from build123d import *

# Parameters (mm, degrees)
SKETCH1_W           = 22.5
SKETCH1_H           = 12.2
BOSS_EXTRUDE1_DEPTH = 22.3
SKETCH2_W           = 12.2
SKETCH2_H           = 2.5
BOSS_EXTRUDE2_DEPTH = 5
CUT_EXTRUDE1_DEPTH  = 28.554396191
SKETCH5_R           = 6.1
BOSS_EXTRUDE3_DEPTH = 4.25
SKETCH6_R           = 2.5
BOSS_EXTRUDE4_DEPTH = 2


with BuildPart() as part:
    # Sketch1 → Boss-Extrude1 (new body)
    with BuildSketch(Plane(origin=(0, 0, 0), x_dir=(1, 0, 0), z_dir=(0, 1, 0))):
        with Locations((3.369036145, -0.994939759)):
            Rectangle(SKETCH1_W, SKETCH1_H)
    extrude(amount=BOSS_EXTRUDE1_DEPTH)

    # Sketch2 → Boss-Extrude2 (add)
    with BuildSketch(Plane(origin=(14.619036145, 0, 0), x_dir=(0, 0, -1), z_dir=(1, 0, 0))):
        with Locations((-0.994939759, 16.75)):
            Rectangle(SKETCH2_W, SKETCH2_H)
    boss_extrude2 = extrude(amount=BOSS_EXTRUDE2_DEPTH)

    # Sketch3 → Cut-Extrude1 (cut, through all)
    with BuildSketch(Plane(origin=(0, 18, 0), x_dir=(1, 0, 0), z_dir=(0, 1, 0))):
        with BuildLine():
            Line((18.271664089, -0.444939759), (19.619036145, -0.444939759))
            Line((19.619036145, -0.444939759), (19.619036145, -1.544939759))
            Line((19.619036145, -1.544939759), (18.271664089, -1.544939759))
            ThreePointArc((18.271664089, -1.544939759), (16.219036145, -0.994939759), (18.271664089, -0.444939759))
        make_face()
    cut_extrude1 = extrude(amount=-CUT_EXTRUDE1_DEPTH, mode=Mode.SUBTRACT)

    # Mirror1: Boss-Extrude2, Cut-Extrude1 across plane
    add(boss_extrude2.mirror(Plane(origin=(3.369036145, 0, 0), x_dir=(0, 0, 1), z_dir=(1, 0, 0))))
    add(cut_extrude1.mirror(Plane(origin=(3.369036145, 0, 0), x_dir=(0, 0, 1), z_dir=(1, 0, 0))), mode=Mode.SUBTRACT)

    # Sketch5 → Boss-Extrude3 (add)
    with BuildSketch(Plane(origin=(0, 22.3, 0), x_dir=(1, 0, 0), z_dir=(0, 1, 0))):
        with Locations(Location((8.519036145, -0.994939759, 0), (0, 0, 270))):
            Circle(SKETCH5_R)
    extrude(amount=BOSS_EXTRUDE3_DEPTH)

    # Sketch6 → Boss-Extrude4 (add)
    with BuildSketch(Plane(origin=(0, 26.55, 0), x_dir=(1, 0, 0), z_dir=(0, 1, 0))):
        with Locations(Location((8.519036145, -0.994939759, 0), (0, 0, 270))):
            Circle(SKETCH6_R)
    extrude(amount=BOSS_EXTRUDE4_DEPTH)


solid = part.part
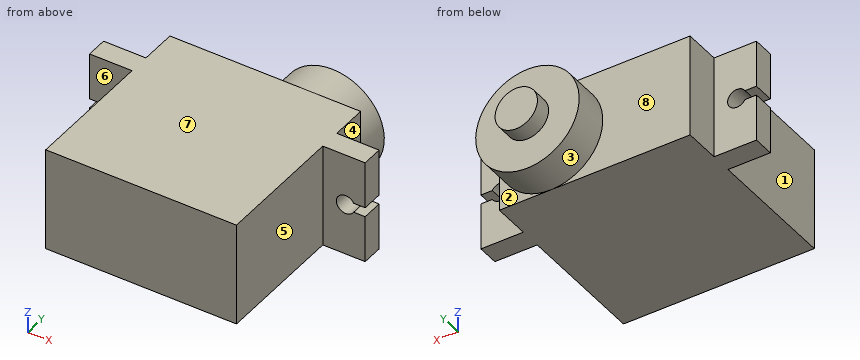
Part model, mm, in its own coordinate system. Face numbers are marked on the shaded views. A direction names the side the tool comes from. Coordinates: 2 decimals unless noted, no trailing zeros. Loops run counter-clockwise (first coordinate to the right, second up) from the corner with the lowest first, then second, coordinate; pieces in that order, holes last. Notation, with made-up numbers: M 28.5,17.5 L 63.5,17.5 A20 cw 63.5,40.5 Z; hole C -27.5,51.25 d11. An arc over 180 degrees is marked long. Use a Markdown table: item, result. Add a question column.
Q1. Cut at D-D (z = 4). Write the cut outline in (x, y), and give its area (3 significant figures).
Q2. Pin check, flat tips, straight feed: P1, Ø1.5, axis at x = 16.5, z = 1.5, coming from the +Y side; P2, Ø6, axis at y = 14.5, z = 4, coming from the +X side; P3, Ø1.5, axis at x = 1.5, z = 1, coming from the +Y side; P4, Ø5.5, axis at x = 18, z = -1.5, coming from the -Y side. Stop position of each tip, or through.
Q3. Cut at B-B (z = -3.5). Write the cut outline in (x, y).
Q4. Mould opens along Y. For the marked faces 6, 7 and 8 say: +Y half, -Y half, draft (parallel to the pull), parting line (faces both ways), or undercut.
Q5. Which spindle directions (+Z, -Z, +X, -X, +Y, -Y) get a long thin tool onto all of the face, cutting with end or side? Do the marked faces 1, 2, 3, 4 and 5. Say none if no direction does.
Q6. Cut at A-A (x = -8.5). Write the cut outline in (y, z).
Q7. Probe L1, parallel to Y at x = -7.5, z = -1.5; L2, parallel to X at y = 13.75, z = 2.75; L3, parallel to Y at x = -9, z = -1.5. List the from-to ranges inside material, lowest first.
Q8. Cut at C-C (y = 10). Write the cut outline in (x, z), and give its area (4 significant figures).
Worked out:
| question | item | result |
|---|---|---|
| 1 | outline | M -12.88,15.5 L -7.88,15.5 L -7.88,0 L 14.62,0 L 14.62,15.5 L 19.62,15.5 L 19.62,18 L 14.62,18 L 14.62,22.3 L 13.83,22.3 L 13.83,26.55 L 3.21,26.55 L 3.21,22.3 L -7.88,22.3 L -7.88,18 L -12.88,18 Z |
| 1 | area | 572 mm2 |
| 2 | P1 | stops at y = 18 |
| 2 | P2 | stops at x = 19.62 |
| 2 | P3 | stops at y = 22.3 |
| 2 | P4 | stops at y = 15.5 |
| 3 | outline | M -12.88,15.5 L -7.88,15.5 L -7.88,0 L 14.62,0 L 14.62,15.5 L 19.62,15.5 L 19.62,18 L 14.62,18 L 14.62,22.3 L 12.64,22.3 L 12.64,26.55 L 4.4,26.55 L 4.4,22.3 L -7.88,22.3 L -7.88,18 L -12.88,18 Z |
| 4 | face 6 | -Y half |
| 4 | face 7 | draft |
| 4 | face 8 | +Y half |
| 5 | face 1 | +Z, -Z, -X, -Y |
| 5 | face 2 | -Z, +X, +Y |
| 5 | face 3 | +Y |
| 5 | face 4 | +Z, -Z, +X, +Y |
| 5 | face 5 | +Z, -Z, +X, -Y |
| 6 | outline | M 15.5,-5.11 L 18,-5.11 L 18,7.09 L 15.5,7.09 Z |
| 7 | L1 | y = 0 to 22.3 |
| 7 | L2 | x = -7.88 to 14.62 |
| 7 | L3 | y = 15.5 to 18 |
| 8 | outline | M -7.88,-5.11 L 14.62,-5.11 L 14.62,7.09 L -7.88,7.09 Z |
| 8 | area | 274.5 mm2 |
